Work out the finished part from the listing and answer in its coordinate system (mm). Face numbers are marked on the shaded views. Give positions to 0.01 mm unless a question says otherwise; leave off trailing zeros. Order: outer loops, then holes, each group sorted by start corner. A loop starts at its lowest first (then second) coordinate and runs counter-clockwise, first axis right, second up.
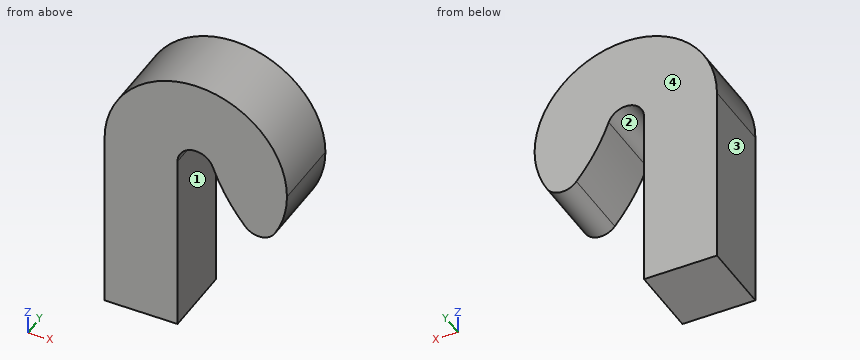
```python
from build123d import *

# Parameters (mm, degrees)
F0_W     = 2
F0_H     = 5
F1_DEPTH = 2
F2_R     = 5
F3_R     = 0.5


with BuildPart() as f1:
    # F0 (on Front) → F1 (new body)
    with BuildSketch(Plane.XZ):
        with Locations((1, 2.5)):
            Rectangle(F0_W, F0_H)
        with BuildLine():
            ThreePointArc((5, 5), (2.5, 7.5), (0, 5))
            Line((0, 5), (2, 5))
            ThreePointArc((2, 5), (2.5, 5.5), (3, 5))
            Line((3, 5), (5, 5))
        make_face()
        with BuildLine():
            ThreePointArc((4.272967, 3.237449), (4.811106, 4.046695), (5, 5))
            Line((5, 5), (3, 5))
            ThreePointArc((3, 5), (2.962221, 4.809339), (2.854593, 4.64749))
            Line((2.854593, 4.64749), (4.272967, 3.237449))
        make_face()
    extrude(amount=F1_DEPTH)

    # F2
    f2_edges = [f1.edges().sort_by_distance(p)[0] for p in [
        (2.854593, -1, 4.64749),
    ]]
    fillet(f2_edges, radius=F2_R)

    # F3
    f3_edges = [f1.edges().sort_by_distance(p)[0] for p in [
        (4.272967, -1, 3.237449),
    ]]
    fillet(f3_edges, radius=F3_R)


solid = f1.part
```
1. Straight lines are drawn through the part: probe 1 along X at (y, z) = (-0.45, 4.5); probe 2 along X at (y, z) = (-0.75, 2.25); probe 3 along Z at (x, y) = (2.5, -0.65). For each, find the intervals that lie inside material, in ascending order.
Findings below:
probe 1: x = 0 to 2, 3.28 to 4.95
probe 2: x = 0 to 2
probe 3: z = 5.5 to 7.5
2. Given P1, Ø0.6, axis at y = -0.5, z = 1.5, coming from the +X side, flat-ended and moving along its own axis, determine where the tip first touches the part or whether it passes through.
Findings below:
P1: stops at x = 2
3. The part is cut by section A-A (x = 2.5). Write down the section's boundary in (y, z).
Findings below:
outline: (-2, 5.5) - (0, 5.5) - (0, 7.5) - (-2, 7.5) - close
4. The part is cut by section B-B (z = 0.5). Write down the section's boundary in (x, y), then the cut area to 3 significant figures.
Findings below:
outline: (0, -2) - (2, -2) - (2, 0) - (0, 0) - close
area: 4.00 mm2
5. The mould has two halves that part along X. Classify the marked faces 1, 2, 3 and 4: pulls with the +X half, pulls with the -X half, needs draft (parallel to the pull), parting line crosses it, or undercut.
Findings below:
face 1: undercut
face 2: undercut
face 3: pulls with the -X half
face 4: needs draft
